```python
from build123d import *

# Parameters (mm, degrees)
F0_W     = 50
F0_H     = 80
F0_R     = 2.75
F1_DEPTH = 10
F3_DEPTH = 50.001
F4_R     = 5


with BuildPart() as f1:
    # F0 (on Top) → F1 (new body)
    with BuildSketch(Plane.XY):
        Rectangle(F0_W, F0_H)
        with Locations((-10, 0)):
            Circle(F0_R, mode=Mode.SUBTRACT)
        with Locations((10, 0)):
            Circle(F0_R, mode=Mode.SUBTRACT)
    extrude(amount=F1_DEPTH)

    # F2 (on face) → F3 (cut, through all)
    with BuildSketch(Plane.YZ.offset(25)):
        with BuildLine():
            ThreePointArc((40, 5), (20.1556440913, 1.2548449991), (-5.632e-07, 0))
            Line((-5.632e-07, 0), (40, 0))
            Line((40, 0), (40, 5))
        make_face()
        with BuildLine():
            ThreePointArc((-5.632e-07, 0), (-20.1556446502, 1.254845069), (-40, 5))
            Line((-40, 5), (-40, 0))
            Line((-40, 0), (-5.632e-07, 0))
        make_face()
    extrude(amount=-F3_DEPTH, mode=Mode.SUBTRACT)

    # F4
    f4_edges = [f1.edges().sort_by_distance(p)[0] for p in [
        (25, -40, 7.5),
        (-25, -40, 7.5),
        (25, 40, 7.5),
        (-25, 40, 7.5),
    ]]
    fillet(f4_edges, radius=F4_R)


solid = f1.part
```
Verification items for the finished model (mm, model axes). Round coordinates to 2 decimals unless told otherwise and drop trailing zeros. Write each loop counter-clockwise with the first axis right and the second up, starting at its lowest first coordinate (ties: lowest second). Pieces come first, ordered by that corner, then holes. Notation, with made-up numbers: (-31, 53.25) - (7, 53.25) arc R8 cw to (7, 58.25) - close; hole circle Ø7 at (70.5, 87.5). An arc over 180 degrees is marked (long way). Answer as a JSON object with one key per item and string values. Group by question number.
Q1. Mould release check, pull along Y, two halves, no side actions. Record for faces 1 (the cylindrical face through (-24, -38, 7)), 2 (the cylindrical face through (23, 39, 7)), 3 (the flat face through (25, 0, 6)), 4 (the cylindrical face through (12.54, -1.05, 4.93)): released by +Y, released by -Y, zero draft, split by the parting line, or undercut.
Q2. Section check A-A, the plane z = 8.5. Enter the section's corners in (x, y), plus the area to 3 significant figures.
Q3. Go/stop test with flat-tipped pins: pin 1 Ø10 at (x, y) = (-11, -8) entering from -Z; pin 2 Ø6 at (x, y) = (-16.5, 16.5) entering from -Z. Record where each tip stops, or that it passes through.
Q4. Thickness scan on line 1 (X direction, y = 0, z = 4); line 2 (Y direction, x = -10, z = 7.5); line 3 (X direction, y = 1, z = 8). Record the ranges inside material, lowest first.
Q5. Section check C-C, the plane y = -1. Enter the section's corners in (x, z), plus the area to 3 significant figures.
Q6. Section check B-B, the plane x = -10. Enter the section's corners in (y, z), plus the area to 3 significant figures.
Q7. Section check D-D, the plane x = -18. Enter the section's corners in (y, z).
Found:
{
 "1": {"face 1": "released by -Y", "face 2": "released by +Y", "face 3": "zero draft", "face 4": "undercut"},
 "2": {"outline": "(-25, -35) arc R5 ccw to (-20, -40) - (20, -40) arc R5 ccw to (25, -35) - (25, 35) arc R5 ccw to (20, 40) - (-20, 40) arc R5 ccw to (-25, 35) - close; hole circle Ø5.5 at (-10, 0); hole circle Ø5.5 at (10, 0)", "area": "3,930 mm^2"},
 "3": {"pin 1": "stops at z = 0.03", "pin 2": "stops at z = 0.56"},
 "4": {"line 1": "x = -25 to -12.75, -7.25 to 7.25, 12.75 to 25", "line 2": "y = -40 to -2.75, 2.75 to 40", "line 3": "x = -25 to -12.56, -7.44 to 7.44, 12.56 to 25"},
 "5": {"outline": "(-25, 0) - (-12.56, 0) - (-12.56, 10) - (-25, 10) - close; (-7.44, 0) - (7.44, 0) - (7.44, 10) - (-7.44, 10) - close; (12.56, 0) - (25, 0) - (25, 10) - (12.56, 10) - close", "area": "397 mm^2"},
 "6": {"outline": "(-40, 5) arc R162.5 ccw to (-2.75, 0.02) - (-2.75, 10) - (-40, 10) - close; (2.75, 0.02) arc R162.5 ccw to (40, 5) - (40, 10) - (2.75, 10) - close", "area": "613 mm^2"},
 "7": {"outline": "(-40, 5) arc R162.5 ccw to (40, 5) - (40, 10) - (-40, 10) - close"}
}
